```python
from build123d import *

# Parameters (mm, degrees)
BOSS_EXTRUDE2_DEPTH = 25.4
SKETCH2_R           = 7.1247
CUT_EXTRUDE1_DEPTH  = 25.4
SKETCH2_3_R         = 7.1247
CUT_EXTRUDE2_DEPTH  = 25.4
SKETCH2_4_R         = 7.1247
CUT_EXTRUDE3_DEPTH  = 25.4
SKETCH2_5_R         = 7.1247
CUT_EXTRUDE4_DEPTH  = 25.4
SKETCH2_6_R         = 7.1247
CUT_EXTRUDE5_DEPTH  = 25.4
SKETCH2_7_R         = 7.1247
CUT_EXTRUDE6_DEPTH  = 25.4
SKETCH2_8_R         = 7.1247
CUT_EXTRUDE7_DEPTH  = 25.4
SKETCH2_9_R         = 7.1247
CUT_EXTRUDE8_DEPTH  = 25.4
SKETCH2_10_R        = 7.1247
CUT_EXTRUDE9_DEPTH  = 25.4
SKETCH2_11_R        = 7.1247
CUT_EXTRUDE10_DEPTH = 25.4


with BuildPart() as part:
    # Pedal Box Floor → Boss-Extrude2 (new body)
    with BuildSketch(Plane.XY):
        Polygon((0, -126.908753769), (-469.9, -123.556557293), (-469.9, 123.556557293), (0, 126.908753769), align=None)
    extrude(amount=BOSS_EXTRUDE2_DEPTH)

    # Sketch2 → Cut-Extrude1 (cut)
    with BuildSketch(Plane.XY):
        with Locations((-235.026595282, 107.199301857)):
            Circle(SKETCH2_R)
    extrude(amount=CUT_EXTRUDE1_DEPTH, mode=Mode.SUBTRACT)

    # Sketch2<3> → Cut-Extrude2 (cut)
    with BuildSketch(Plane.XY):
        with Locations((-18.034, 0)):
            Circle(SKETCH2_3_R)
    extrude(amount=CUT_EXTRUDE2_DEPTH, mode=Mode.SUBTRACT)

    # Sketch2<4> → Cut-Extrude3 (cut)
    with BuildSketch(Plane.XY):
        with Locations((-451.866, 0)):
            Circle(SKETCH2_4_R)
    extrude(amount=CUT_EXTRUDE3_DEPTH, mode=Mode.SUBTRACT)

    # Sketch2<5> → Cut-Extrude4 (cut)
    with BuildSketch(Plane.XY):
        with Locations((-235.026595282, -107.200076916)):
            Circle(SKETCH2_5_R)
    extrude(amount=CUT_EXTRUDE4_DEPTH, mode=Mode.SUBTRACT)

    # Sketch2<6> → Cut-Extrude5 (cut)
    with BuildSketch(Plane.XY):
        with Locations((-273.05, -69.85)):
            Circle(SKETCH2_6_R)
    extrude(amount=CUT_EXTRUDE5_DEPTH, mode=Mode.SUBTRACT)

    # Sketch2<7> → Cut-Extrude6 (cut)
    with BuildSketch(Plane.XY):
        with Locations((-184.15, -69.85)):
            Circle(SKETCH2_7_R)
    extrude(amount=CUT_EXTRUDE6_DEPTH, mode=Mode.SUBTRACT)

    # Sketch2<8> → Cut-Extrude7 (cut)
    with BuildSketch(Plane.XY):
        with Locations((-95.25, -69.85)):
            Circle(SKETCH2_8_R)
    extrude(amount=CUT_EXTRUDE7_DEPTH, mode=Mode.SUBTRACT)

    # Sketch2<9> → Cut-Extrude8 (cut)
    with BuildSketch(Plane.XY):
        with Locations((-273.05, 69.85)):
            Circle(SKETCH2_9_R)
    extrude(amount=CUT_EXTRUDE8_DEPTH, mode=Mode.SUBTRACT)

    # Sketch2<10> → Cut-Extrude9 (cut)
    with BuildSketch(Plane.XY):
        with Locations((-184.15, 69.85)):
            Circle(SKETCH2_10_R)
    extrude(amount=CUT_EXTRUDE9_DEPTH, mode=Mode.SUBTRACT)

    # Sketch2<11> → Cut-Extrude10 (cut)
    with BuildSketch(Plane.XY):
        with Locations((-95.25, 69.85)):
            Circle(SKETCH2_11_R)
    extrude(amount=CUT_EXTRUDE10_DEPTH, mode=Mode.SUBTRACT)


solid = part.part
```
Geometry: final body of the model. Coordinates: model frame, mm. Coordinates: 2 decimals unless noted, no trailing zeros. Order: outer loops, then holes, each group sorted by start corner. A loop starts at its lowest first (then second) coordinate and runs counter-clockwise, first axis right, second up. Notation, with made-up numbers: (-24, 86) -> (3, 86) arc R27 cw to (3, 113) -> close; hole circle Ø11 at (-9, -2.75). An arc over 180 degrees is marked (long way). Write each question's results on one line, items separated by ' | '. Start each with the question number.
1) Cut plane B-B, the plane x = -273. Output: boundary loops of the cut face in (y, z), and give its area (3 significant figures).
2) Cut plane A-A, the plane y = -69.85. Output: boundary loops of the cut face in (x, z).
3) Cut plane C-C, the plane z = 4.75. State how many separate pieces and enclosed holes the cut face has, and give its area (3 significant figures).
4) First-contact query: pin 1 (23 mm diameter, centred on x = -95.25, y = 69.85, fed in from +Z); pin 2 (11.5 mm diameter, centred on x = -273.05, y = -69.85, fed in from +Z); pin 3 (12 mm diameter, centred on x = -67.5, z = 11.5, fed in from +Y). Flat tips, straight axial feed; report the tip coordinate or a pass-through.
5) Mould query, pull axis X, two halves, no side actions, for faces 1 (the cylindrical face through (-242.144, 107.513, 12.522)), 2 (the flat face through (-469.9, -2, 13)), 3 (the flat face through (-232, 2, 25.4)). Classes: released by +X, released by -X, zero draft, split by the parting line, or undercut.
6) Material intervals for line 1 along X through (y, z) = (69, 19.25); line 2 along Y through (x, z) = (-90.5, 5); line 3 along Y through (x, z) = (-273.05, 11.25), sorted ascending.
7) Cut plane D-D, the plane x = -95.25. Output: boundary loops of the cut face in (y, z).
Checks:
1) outline: (-124.96, 0) -> (-76.97, 0) -> (-76.97, 25.4) -> (-124.96, 25.4) -> close; (-62.73, 0) -> (62.73, 0) -> (62.73, 25.4) -> (-62.73, 25.4) -> close; (76.97, 0) -> (124.96, 0) -> (124.96, 25.4) -> (76.97, 25.4) -> close | area: 5,620 mm^2
2) outline: (-469.9, 0) -> (-280.17, 0) -> (-280.17, 25.4) -> (-469.9, 25.4) -> close; (-265.93, 0) -> (-191.27, 0) -> (-191.27, 25.4) -> (-265.93, 25.4) -> close; (-177.03, 0) -> (-102.37, 0) -> (-102.37, 25.4) -> (-177.03, 25.4) -> close; (-88.13, 0) -> (0, 0) -> (0, 25.4) -> (-88.13, 25.4) -> close
3) separate pieces: 1 | enclosed holes: 10 | area: 116,000 mm^2
4) pin 1: z = 25.4 | pin 2: through | pin 3: y = 126.47
5) face 1: undercut | face 2: released by -X | face 3: zero draft
6) line 1: -469.9 to -280.12, -265.98 to -191.22, -177.08 to -102.32, -88.18 to 0 | line 2: -126.26 to -75.16, -64.54 to 64.54, 75.16 to 126.26 | line 3: -124.96 to -76.97, -62.73 to 62.73, 76.97 to 124.96
7) outline: (-126.23, 0) -> (-76.97, 0) -> (-76.97, 25.4) -> (-126.23, 25.4) -> close; (-62.73, 0) -> (62.73, 0) -> (62.73, 25.4) -> (-62.73, 25.4) -> close; (76.97, 0) -> (126.23, 0) -> (126.23, 25.4) -> (76.97, 25.4) -> close
